Design review of the part shown in the three views and the two pictorial views. Dimensions are in mm from the part's minimum x, y and z. A direction names the side the tool comes from. Coordinates: 2 decimals unless noted, no trailing zeros. Loops run counter-clockwise (first coordinate to the right, second up) from the corner with the lowest first, then second, coordinate; pieces in that order, holes last. Notation, with made-up numbers: M -7.5,-29.5 L 50.5,-29.5 A25 cw 50.5,-17.5 Z; hole C -4,-17 d7. An arc over 180 degrees is marked long. Put each result on its own line as item: value. Start each with the question number.
(1) Take a section at C-C, the plane z = 23. Give the boundary of the cut face in (x, y), then the cut area to 3 significant figures.
(2) For the marked faces 1 and 2, list the 3-axis set-ups (+Z, -Z, +X, -X, +Y, -Y) from which the entire face can be reached by the end or side of a thin tool; tool diameter is ignored.
(3) Clearance check with flat-ended pins moving along their axes: pin 1 (4 mm diameter, centred on x = 3.5, y = 21.5, fed in from -Z); pin 2 (1 mm diameter, centred on y = 21.5, z = 19.5, fed in from -X). State where each tip first meets the part, or that it passes through.
(4) Take a section at B-B, the plane x = 2.5. Give the boundary of the cut face in (y, z), then the cut area to 3 significant figures.
(5) For probe 1 along X at (y, z) = (13, 33); probe 2 along Z at (x, y) = (2.5, 3.5); probe 3 along Z at (x, y) = (8, 6.75), list the stretches that pass through material, from the lowest coordinate up. Write a range as [from, to].
(6) Take a section at A-A, the plane y = 14. Give the boundary of the cut face in (x, z).
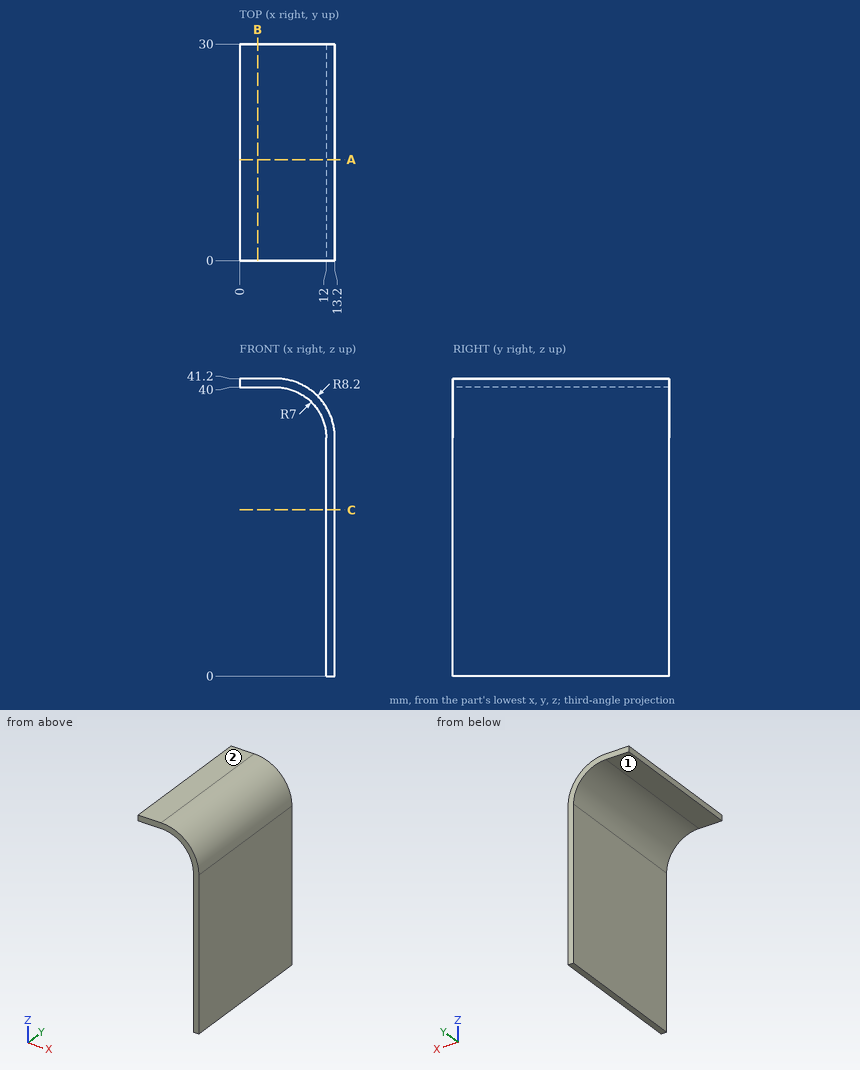
Computed values:
1. outline: M 12,0 L 13.2,0 L 13.2,30 L 12,30 Z
1. area: 36.0 mm^2
2. face 1: -Z, -X, +Y, -Y
2. face 2: +Z, +X, -X, +Y, -Y
3. pin 1: stops at z = 39.98
3. pin 2: stops at x = 12
4. outline: M 0,40 L 30,40 L 30,41.2 L 0,41.2 Z
4. area: 36.0 mm^2
5. probe 1: x = [12, 13.2]
5. probe 2: z = [40, 41.2]
5. probe 3: z = [39.32, 40.63]
6. outline: M 0,40 L 5,40 A7 cw 12,33 L 12,0 L 13.2,0 L 13.2,33 A8.2 ccw 5,41.2 L 0,41.2 Z
